from build123d import *

# Parameters (mm, degrees)
F1_DEPTH = 25.4


with BuildPart() as f1:
    # F0 (on Front) → F1 (new body)
    with BuildSketch(Plane.XZ):
        with BuildLine():
            ThreePointArc((70.111157, -29.528858), (64.82074, 1.313272), (69.386698, 32.270945))
            ThreePointArc((69.386698, 32.270945), (51.992809, 39.03154), (34.59892, 32.270945))
            ThreePointArc((34.59892, 32.270945), (29.893964, 1.244372), (36.041575, -29.528858))
            ThreePointArc((36.041575, -29.528858), (53.076366, -35.966931), (70.111157, -29.528858))
        make_face()
        with BuildLine():
            ThreePointArc((101.791199, 27.068468), (84.635881, 23.733368), (69.386698, 32.270945))
            ThreePointArc((69.386698, 32.270945), (64.82074, 1.313272), (70.111157, -29.528858))
            ThreePointArc((70.111157, -29.528858), (85.560524, -24.101311), (101.791199, -26.270727))
            ThreePointArc((101.791199, -26.270727), (98.099114, 0.39887), (101.791199, 27.068468))
        make_face()
        with BuildLine():
            ThreePointArc((36.041575, -29.528858), (29.893964, 1.244372), (34.59892, 32.270945))
            ThreePointArc((34.59892, 32.270945), (16.047725, 29.245195), (0, 39.03154))
            Line((0, 39.03154), (-53.967841, 39.03154))
            ThreePointArc((-53.967841, 39.03154), (-60.466973, 1.200982), (-50.878648, -35.966931))
            Line((-50.878648, -35.966931), (0, -35.966931))
            ThreePointArc((0, -35.966931), (16.76772, -25.732983), (36.041575, -29.528858))
        make_face()
        with BuildLine():
            ThreePointArc((129.847508, 27.068468), (115.819353, 30.70991), (101.791199, 27.068468))
            ThreePointArc((101.791199, 27.068468), (98.099114, 0.39887), (101.791199, -26.270727))
            ThreePointArc((101.791199, -26.270727), (115.819353, -29.729842), (129.847508, -26.270727))
            ThreePointArc((129.847508, -26.270727), (130.654455, -20.145006), (129.847508, -14.019285))
            ThreePointArc((129.847508, -14.019285), (128.08968, 0.688918), (129.847508, 15.397122))
            ThreePointArc((129.847508, 15.397122), (130.317745, 21.232795), (129.847508, 27.068468))
        make_face()
        with BuildLine():
            ThreePointArc((152.453851, 15.397122), (141.150679, 15.689305), (129.847508, 15.397122))
            ThreePointArc((129.847508, 15.397122), (128.08968, 0.688918), (129.847508, -14.019285))
            ThreePointArc((129.847508, -14.019285), (141.150679, -14.335005), (152.453851, -14.019285))
            ThreePointArc((152.453851, -14.019285), (154.9497, 0.688918), (152.453851, 15.397122))
        make_face()
    extrude(amount=F1_DEPTH)


solid = f1.part
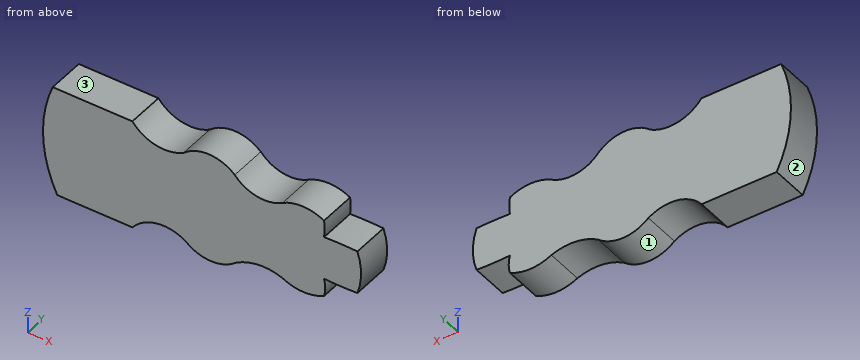
Could you check a few things on this model? Use its own coordinates, in mm. Face numbers are marked on the shaded views. Give positions to 0.01 mm unless a question says otherwise; leave off trailing zeros. Order: outer loops, then holes, each group sorted by start corner. A loop starts at its lowest first (then second) coordinate and runs counter-clockwise, first axis right, second up. Notation, with made-up numbers: (24.25, 3.5) - (47.25, 3.5) arc R23 cw to (47.25, 16.5) - close; hole circle Ø10 at (-13.5, 69.25). An arc over 180 degrees is marked (long way). One line per question, with ' | ' between items. Start each with the question number.
Item 1: I want a section at A-A on y = -19. Write out the boundary of the cut face in (x, z) (1 decimal), then the cut area to 3 significant figures.
Item 2: I want a section at C-C on x = 111. Write out the boundary of the cut face in (y, z).
Item 3: I need wall thicknesses on probe 1 along X at (y, z) = (-11.5, 26.5); probe 2 along Z at (x, y) = (141, -21); probe 3 along Z at (x, y) = (33.5, -4.25). Which ranges of each line are inside material? Lowest first, please. Write a range as [from, to].
Item 4: I'm going to push flat-ended pins straight in: pin 1 Ø3 at (x, y) = (30.5, -12.5) entering from +Z; pin 2 Ø1.5 at (x, z) = (18, 31.5) entering from +Y; pin 3 Ø10 at (x, y) = (76, -3) entering from -Z; pin 4 Ø12 at (x, y) = (80.5, -10) entering from -Z. Where does each tip first touch, or does it pass through?
Item 5: Thinking about a two-plate mould opening in X: for the marked faces 1, 2 and 3, which applies, pulls with the +X half, pulls with the -X half, needs draft (parallel to the pull), parting line crosses it, or undercut?
Item 6: I want a section at B-B on z = 19. Write out the boundary of the cut face in (x, y).
Verdict:
1) outline: (-54, 39) arc R91.5 ccw to (-50.9, -36) - (0, -36) arc R27.1 cw to (36, -29.5) arc R25.8 ccw to (70.1, -29.5) arc R35.1 cw to (101.8, -26.3) arc R30.2 ccw to (129.8, -26.3) arc R23.7 ccw to (129.8, -14) arc R202.5 ccw to (152.5, -14) arc R44.6 ccw to (152.5, 15.4) arc R218.8 ccw to (129.8, 15.4) arc R36.4 ccw to (129.8, 27.1) arc R28.8 ccw to (101.8, 27.1) arc R25.4 cw to (69.4, 32.3) arc R25.8 ccw to (34.6, 32.3) arc R27.1 cw to (0, 39) - close | area: 12,800 mm^2
2) outline: (-25.4, -29.34) - (0, -29.34) - (0, 30.3) - (-25.4, 30.3) - close
3) probe 1: [-57.97, 76.52], [100.8, 129.94] | probe 2: [-14.33, 15.69] | probe 3: [-28.1, 31.68]
4) pin 1: z = 30.97 | pin 2: through | pin 3: z = -28.97 | pin 4: z = -27.12
5) face 1: undercut | face 2: pulls with the -X half | face 3: needs draft
6) outline: (-59.46, -25.4) - (130.25, -25.4) - (130.25, 0) - (-59.46, 0) - close
